Geometry: see drawing. Coordinates: mm, zero at the bounding-box minimum. A direction names the side the tool comes from. Give positions to 0.01 mm unless a question says otherwise; leave off trailing zeros. Write each loop counter-clockwise with the first axis right and the second up, starting at its lowest first coordinate (ties: lowest second). Pieces come first, ordered by that corner, then holes.
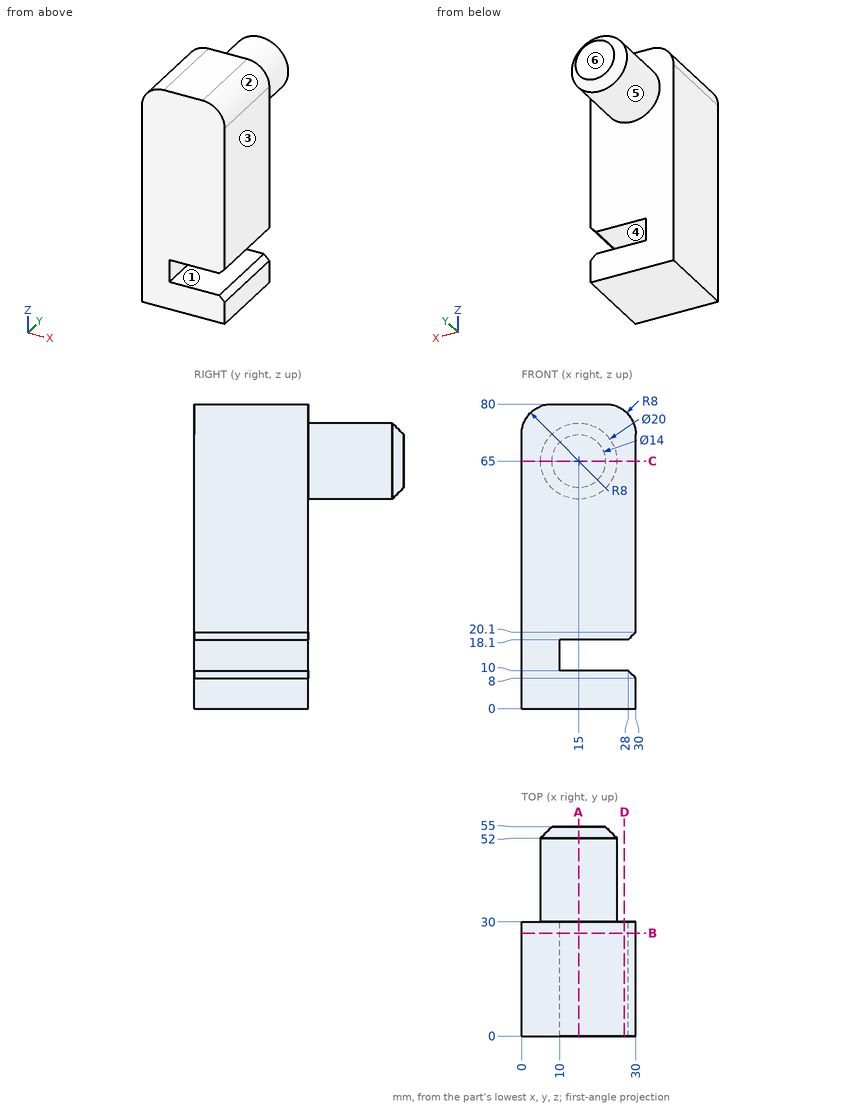
Q1. Section B-B, the plane y = 27. Return the cut outline in (x, z), then the cut area to 3 significant figures.
Q2. Section C-C, the plane z = 65. Return the cut outline in (x, y), then the cut area to 3 significant figures.
Q3. Pin query (flat end, axial travel): pin 1 (4 mm diameter, centred on x = 21, y = 39.5, fed in from +Z); pin 2 (4 mm diameter, centred on x = 15, y = 36.5, fed in from -Z); pin 3 (4 mm diameter, centred on y = 15, z = 14.5, fed in from +X). Return the tip coordinate at first contact, or that it passes through.
Q4. Access query for the marked faces 4, 5 and 6. Directions: +Z, -Z, +X, -X, +Y, -Y. A direction counts if a zero-diameter tool reaches every point of the face in a straight line with its end or side. Return the directions, or none.
Q5. Section A-A, the plane x = 15. Return the cut outline in (y, z), then the cut area to 3 significant figures.
Q6. Mould query, pull axis Z, two halves, no side actions, for the marked faces 1, 2 and 3. Classes: +Z half, -Z half, draft (parallel to the pull), parting line (faces both ways), or undercut.
Q7. Material intervals for line 1 along Z through (x, y) = (18, 4); line 2 along X through (y, z) = (6.5, 12); line 3 along Y through (x, z) = (6.5, 76), sorted ascending.
Q8. Section D-D, the plane x = 27. Return the cut outline in (y, z) (3 decimals), then the cut area to 3 significant figures.
Solutions:
1. outline: (0, 0) - (30, 0) - (30, 8) - (28, 10) - (10, 10) - (10, 18.1) - (28, 18.1) - (30, 20.1) - (30, 72) arc R8 ccw to (22, 80) - (8, 80) arc R8 ccw to (0, 72) - close
1. area: 2,210 mm2
2. outline: (0, 0) - (30, 0) - (30, 30) - (25, 30) - (25, 52) - (22, 55) - (8, 55) - (5, 52) - (5, 30) - (0, 30) - close
2. area: 1,390 mm2
3. pin 1: stops at z = 74.17
3. pin 2: stops at z = 55
3. pin 3: stops at x = 10
4. face 4: +X, +Y, -Y
4. face 5: +Y
4. face 6: +Z, -Z, +X, -X, +Y
5. outline: (0, 0) - (30, 0) - (30, 10) - (0, 10) - close; (0, 18.1) - (30, 18.1) - (30, 55) - (52, 55) - (55, 58) - (55, 72) - (52, 75) - (30, 75) - (30, 80) - (0, 80) - close
5. area: 2,650 mm2
6. face 1: undercut
6. face 2: +Z half
6. face 3: draft
7. line 1: z = 0 to 10, 18.1 to 80
7. line 2: x = 0 to 10
7. line 3: y = 0 to 30
8. outline: (0, 0) - (30, 0) - (30, 10) - (0, 10) - close; (0, 18.1) - (30, 18.1) - (30, 78.245) - (0, 78.245) - close
8. area: 2,100 mm2
